Design review of the part built by this model. Coordinates are the model's own, in mm. A direction names the side the tool comes from. Round coordinates to 2 decimals unless told otherwise and drop trailing zeros. Loops run counter-clockwise (first coordinate to the right, second up) from the corner with the lowest first, then second, coordinate; pieces in that order, holes last. Notation, with made-up numbers: M 25.5,10 L 69.5,10 A13 ccw 69.5,35 Z; hole C 12,-28 d3. An arc over 180 degrees is marked long. Use a Markdown table: item, result.
Autodesk Inventor part; units mm, degrees
ref_plane "YZ Plane" through (0, 0, 0) normal (1, 0, 0) x (0, 1, 0)
ref_plane "XZ Plane" through (0, 0, 0) normal (0, 1, 0) x (-1, 0, 0)
ref_plane "XY Plane" through (0, 0, 0) normal (0, 0, 1) x (1, 0, 0)
sketch "Sketch1" plane through (0, 0, 0) normal (0, 0, 1) x (1, 0, 0)
  circle A0 centre (0, 0) radius 3.75
  dimension "d0" = 7.5
extrude "Extrusion1" add sketch "Sketch1" along normal blind 16
sketch "Sketch2" plane through (0, 0, 16) normal (0, 0, 1) x (1, 0, 0)
  circle A0 centre (0, 0) radius 3.75
  line L0 (-2.7951, 2.5) -> (2.7951, 2.5)
  dimension "d3" = 2.5
extrude "Extrusion2" cut sketch "Sketch2" against normal through all contours L0 A0 picked at (-0.7066, 2.6978)
sketch "Sketch3" plane through (0, 0, 0) normal (0, 0, -1) x (-1, 0, 0)
  circle A0 centre (0, 0) radius 4
  dimension "d6" = 8
extrude "Extrusion3" add sketch "Sketch3" against normal blind 1
properties material "Stainless Steel"
1. Wall thickness on line 1 along Z through (x, y) = (3.25, 2); line 2 along Y through (x, z) = (2.5, 2.5); line 3 along Y through (x, z) = (1.25, 8): over which ranges is each line inside the solid? List them lowest first. Write a range as from..to.
Check values:
| item | result |
|---|---|
| line 1 | z = 0..1 |
| line 2 | y = -2.8..2.5 |
| line 3 | y = -3.54..2.5 |
2. Take a section at B-B on y = 0. Give the boundary of the cut face in (x, z).
Check values:
| item | result |
|---|---|
| outline | M -4,0 L 4,0 L 4,1 L 3.75,1 L 3.75,16 L -3.75,16 L -3.75,1 L -4,1 Z |
3. Take a section at A-A on x = 0. Give the boundary of the cut face in (y, z).
Check values:
| item | result |
|---|---|
| outline | M -4,0 L 4,0 L 4,1 L 2.5,1 L 2.5,16 L -3.75,16 L -3.75,1 L -4,1 Z |
4. Take a section at C-C on z = 5.5. Give the boundary of the cut face in (x, y).
Check values:
| item | result |
|---|---|
| outline | M -2.8,2.5 A3.75 ccw long 2.8,2.5 Z |
5. Insertion check: pin 1 (1.5 mm diameter, centred on x = -0.5, z = 8, fed in from -Y); pin 2 (1.7 mm diameter, centred on x = 1, z = 12, fed in from +Y); pin 3 (1.5 mm diameter, centred on y = 2, z = 10, fed in from +X). Each pin has a flat end and moves straight along its axis. Give the tip position at first contact, or say it passes through.
Check values:
| item | result |
|---|---|
| pin 1 | stops at y = -3.75 |
| pin 2 | stops at y = 2.5 |
| pin 3 | stops at x = 3.54 |
6. Machinability: for faces 1 (the face through (0.867, -3.905, 0.493)), 2 (the face through (0.12, -3.75, 8.4)), 3 (the face through (0, 2.5, 9)), which of the approach directions +Z, -Z, +X, -X, +Y, -Y give a long, thin tool a straight path to every point of the face, cutting with its end or side? Answer none if there is none.
Check values:
| item | result |
|---|---|
| face 1 | +Z, -Z |
| face 2 | +Z |
| face 3 | +Z, +X, -X, +Y |
